from build123d import *

# Parameters (mm, degrees)
F0_W      = 38
F0_H      = 38
F1_DEPTH  = 9.3
F2_R      = 1.5
F3_DEPTH  = 0.75
F5_DEPTH  = 0.5
F6_W      = 1.1
F6_H      = 0.54
F7_DEPTH  = 0.5
F8_R      = 0.25
F9_W      = 28
F9_H      = 28
F10_DEPTH = 5
F11_SIZE  = 0.5


with BuildPart() as f1:
    # F0 (on Front) → F1 (new body)
    with BuildSketch(Plane.XZ):
        Rectangle(F0_W, F0_H)
    extrude(amount=F1_DEPTH)

    # F2 (on face) → F3 (cut)
    with BuildSketch(Plane.XZ.offset(9.3)):
        with Locations((-16.8, 16.8)):
            Circle(F2_R)
        with Locations((16.8, 16.8)):
            Circle(F2_R)
        with Locations((16.8, -16.8)):
            Circle(F2_R)
        with Locations((-16.8, -16.8)):
            Circle(F2_R)
    extrude(amount=-F3_DEPTH, mode=Mode.SUBTRACT)

    # F4 (on face) → F5 (join)
    with BuildSketch(Plane.XZ.offset(9.3)):
        Polygon((14, 19), (0, 19), (-14, 19), (-14, 13.3), (-14.54, 13.3), (-14.54, 12.2), (-14, 12.2), (-14, 8.2), (-14.54, 8.2), (-14.54, 7.1), (-14, 7.1), (-14, 3.1), (-14.54, 3.1), (-14.54, 2), (-14, 2), (-14, -2), (-14.54, -2), (-14.54, -3.1), (-14, -3.1), (-14, -7.1), (-14.54, -7.1), (-14.54, -8.2), (-14, -8.2), (-14, -12.2), (-14.54, -12.2), (-14.54, -13.3), (-14, -13.3), (-14, -19), (0, -19), (14, -19), (14, -13.3), (14.54, -13.3), (14.54, -12.2), (14, -12.2), (14, -8.2), (14.54, -8.2), (14.54, -7.1), (14, -7.1), (14, -3.1), (14.54, -3.1), (14.54, -2), (14, -2), (14, 2), (14.54, 2), (14.54, 3.1), (14, 3.1), (14, 7.1), (14.54, 7.1), (14.54, 8.2), (14, 8.2), (14, 12.2), (14.54, 12.2), (14.54, 13.3), (14, 13.3), align=None)
    extrude(amount=F5_DEPTH)

    # F6 (on face) → F7 (join)
    with BuildSketch(Plane.XZ.offset(9.8)):
        Polygon((14, 17.2), (14, 19), (-14, 19), (-14, 17.2), (-12.9, 17.2), (-8.6, 17.2), (-7.5, 17.2), (-3.2, 17.2), (-2.1, 17.2), (2.1, 17.2), (3.2, 17.2), (7.5, 17.2), (8.6, 17.2), (12.9, 17.2), align=None)
        with Locations((13.45, 16.93)):
            Rectangle(F6_W, F6_H)
        with Locations((-13.45, 16.93)):
            Rectangle(F6_W, F6_H)
        with Locations((8.05, 16.93)):
            Rectangle(F6_W, F6_H)
        with Locations((-8.05, 16.93)):
            Rectangle(F6_W, F6_H)
        with Locations((2.65, 16.93)):
            Rectangle(F6_W, F6_H)
        with Locations((-2.65, 16.93)):
            Rectangle(F6_W, F6_H)
        with Locations((-13.45, -16.93)):
            Rectangle(F6_W, F6_H)
        Polygon((-12.9, -17.2), (-14, -17.2), (-14, -19), (14, -19), (14, -17.2), (12.9, -17.2), (8.6, -17.2), (7.5, -17.2), (3.2, -17.2), (2.1, -17.2), (-2.1, -17.2), (-3.2, -17.2), (-7.5, -17.2), (-8.6, -17.2), align=None)
        with Locations((-8.05, -16.93)):
            Rectangle(F6_W, F6_H)
        with Locations((13.45, -16.93)):
            Rectangle(F6_W, F6_H)
        with Locations((-2.65, -16.93)):
            Rectangle(F6_W, F6_H)
        with Locations((8.05, -16.93)):
            Rectangle(F6_W, F6_H)
        with Locations((2.65, -16.93)):
            Rectangle(F6_W, F6_H)
    extrude(amount=F7_DEPTH)

    # F8
    f8_edges = [f1.edges().sort_by_distance(p)[0] for p in [
        (-19, -9.3, 0),
        (19, -9.3, 0),
    ]]
    fillet(f8_edges, radius=F8_R)

    # F9 (on face) → F10 (cut)
    with BuildSketch(Plane.XZ):
        Rectangle(F9_W, F9_H)
    extrude(amount=F10_DEPTH, mode=Mode.SUBTRACT)

    # F11
    f11_edges = [f1.edges().sort_by_distance(p)[0] for p in [
        (-14, -2.5, 14),
        (0, -5, 14),
        (-14, -5, 0),
        (14, -2.5, 14),
        (14, -2.5, -14),
        (14, 0, 0),
        (14, -5, 0),
        (-14, -2.5, -14),
        (0, 0, -14),
        (0, -5, -14),
        (0, 0, 14),
        (-14, 0, 0),
    ]]
    chamfer(f11_edges, length=F11_SIZE)


solid = f1.part
Build history of the part. All positions in model axes, mm. A direction names the side the tool comes from. Round coordinates to 2 decimals unless told otherwise and drop trailing zeros. Write each loop counter-clockwise with the first axis right and the second up, starting at its lowest first coordinate (ties: lowest second). Pieces come first, ordered by that corner, then holes. Notation, with made-up numbers: M -24.75,40.25 L 21.25,40.25 A16 cw 21.25,57.25 Z; hole C 64.5,-36 d1. An arc over 180 degrees is marked long. Answer as a JSON object with one key per item and string values. Group by question number.
(1) Drill centre lines: L1, parallel to Z at x = -16.8, y = -8.9; L2, parallel to Z at x = 6, y = -2.75. Where is each one in solid material? Low to high.
(2) Flat gauge pins, fed straight in: pin 1 (10 mm diameter, centred on x = 12, z = 6, fed in from -Y); pin 2 (1.5 mm diameter, centred on x = 16.5, z = -17, fed in from -Y); pin 3 (3.5 mm diameter, centred on x = -17, z = -16, fed in from -Y). Where does each tip first touch, or does it go through?
(3) Which spindle directions (+Z, -Z, +X, -X, +Y, -Y) get a long thin tool onto all of the face, cutting with end or side? Do faces 4 (the flat face through (0, -10.3, -18)), 5 (the flat face through (17, -8.55, -17)), 6 (the flat face through (0, -5, 0)). Say none if no direction does.
(4) Cut at B-B (x = -12). Give the cut face in (y, z), and give its area (3 significant figures).
(5) Cut at A-A (y = -1.75). Give the cut face in (x, z), and give its area (4 significant figures).
(6) Cut at D-D (x = 16). Give the cut face in (y, z).
(7) Cut at C-C (x = -16.8). Give the cut face in (y, z), and give its area (3 significant figures).
(8) Mould opens along X. For faces 1 (the flat face through (0, -5, 19)), 2 (the flat face through (14, -2, 0)), 3 (the flat face through (-14, -10, -17)) say: pulls with the +X half, pulls with the -X half, needs draft (parallel to the pull), parting line crosses it, or undercut.
Responses:
{
 "1": {"L1": "z = -19 to -18.3, -15.3 to 15.3, 18.3 to 19", "L2": "z = -19 to -14, 14 to 19"},
 "2": {"pin 1": "stops at y = -9.8", "pin 2": "stops at y = -8.55", "pin 3": "stops at y = -9.3"},
 "3": {"face 4": "+Z, -Z, +X, -X, -Y", "face 5": "-Y", "face 6": "+Y"},
 "4": {"outline": "M -10.3,-19 L 0,-19 L 0,-14.5 L -0.5,-14 L -4.5,-14 L -5,-13.5 L -5,13.5 L -4.5,14 L -0.5,14 L 0,14.5 L 0,19 L -10.3,19 L -10.3,17.2 L -9.8,17.2 L -9.8,-17.2 L -10.3,-17.2 Z", "area": "234 mm2"},
 "5": {"outline": "M -19,-19 L 19,-19 L 19,19 L -19,19 Z; hole M -14,-13.5 L -13.5,-14 L 13.5,-14 L 14,-13.5 L 14,13.5 L 13.5,14 L -13.5,14 L -14,13.5 Z", "area": "660.5 mm2"},
 "6": {"outline": "M -9.3,-19 L 0,-19 L 0,19 L -9.3,19 L -9.3,18.07 L -8.55,18.07 L -8.55,15.53 L -9.3,15.53 L -9.3,-15.53 L -8.55,-15.53 L -8.55,-18.07 L -9.3,-18.07 Z"},
 "7": {"outline": "M -9.3,-19 L 0,-19 L 0,19 L -9.3,19 L -9.3,18.3 L -8.55,18.3 L -8.55,15.3 L -9.3,15.3 L -9.3,-15.3 L -8.55,-15.3 L -8.55,-18.3 L -9.3,-18.3 Z", "area": "349 mm2"},
 "8": {"face 1": "needs draft", "face 2": "undercut", "face 3": "pulls with the -X half"}
}
